from build123d import *

# Parameters (mm, degrees)
SALIENTE_EXTRUIR1_DEPTH = 15.875
REDONDEO1_R             = 15.875
CORTAR_EXTRUIR1_REACH   = 48.084
CROQUIS2_R              = 9.525
CROQUIS3_R              = 12.7
CORTAR_EXTRUIR2_DEPTH   = 47.084243503
CROQUIS4_R              = 3.2639
CROQUIS4_R_2            = 2.4892
CORTAR_EXTRUIR3_DEPTH   = 47.084243503
REDONDEO2_R             = 2.54
REDONDEO3_R             = 1.27


with BuildPart() as part:
    # Croquis1 → Saliente-Extruir1 (new body)
    with BuildSketch(Plane.XY):
        Polygon((30.48, 0), (-30.48, 0), (-30.48, 6.35), (12.046472996, 38.277805334), (30.48, 6.35), align=None)
    extrude(amount=SALIENTE_EXTRUIR1_DEPTH)

    # Redondeo1
    redondeo1_edges = [part.edges().sort_by_distance(p)[0] for p in [
        (12.046472996, 38.277805334, 7.9375),
    ]]
    fillet(redondeo1_edges, radius=REDONDEO1_R)

    # Croquis2 → Cortar-Extruir1 (cut, up to next)
    with BuildSketch(Plane.XY.offset(15.875), mode=Mode.PRIVATE) as cortar_extruir1_sk1:
        with Locations((7.254003, 16.09860686)):
            Circle(CROQUIS2_R)
    cortar_extruir1_tool1 = extrude(cortar_extruir1_sk1.sketch, amount=-CORTAR_EXTRUIR1_REACH, mode=Mode.PRIVATE) & part.part
    add(cortar_extruir1_tool1.solids().sort_by_distance((7.254003, 16.098607, 15.875))[0], mode=Mode.SUBTRACT)

    # Croquis3 → Cortar-Extruir2 (cut, through all)
    with BuildSketch(Plane.XY.offset(15.875)):
        with Locations((7.254003, 16.09860686)):
            Circle(CROQUIS3_R)
    extrude(amount=-CORTAR_EXTRUIR2_DEPTH, mode=Mode.SUBTRACT)

    # Croquis4 → Cortar-Extruir3 (cut, through all)
    with BuildSketch(Plane.XZ):
        with Locations((-23.8125, 11.43)):
            Circle(CROQUIS4_R)
        with Locations(Location((23.8125, 11.43, 0), (0, 0, 210.56660833))):
            Circle(CROQUIS4_R)
        with Locations((7.254003, 9.525)):
            Circle(CROQUIS4_R_2)
    extrude(amount=-CORTAR_EXTRUIR3_DEPTH, mode=Mode.SUBTRACT)

    # Redondeo2
    redondeo2_edges = [part.edges().sort_by_distance(p)[0] for p in [
        (-30.48, 6.35, 7.9375),
        (30.48, 6.35, 7.9375),
    ]]
    fillet(redondeo2_edges, radius=REDONDEO2_R)

    # Redondeo3
    redondeo3_edges = [part.edges().sort_by_distance(p)[0] for p in [
        (30.48, 0, 7.9375),
        (-30.48, 0, 7.9375),
    ]]
    fillet(redondeo3_edges, radius=REDONDEO3_R)


solid = part.part
Model file for the job. Use its own axes, mm. Round coordinates to 2 decimals unless told otherwise and drop trailing zeros. Loops run counter-clockwise (first coordinate to the right, second up) from the corner with the lowest first, then second, coordinate; pieces in that order, holes last. Notation, with made-up numbers: (26.25, 45) - (68.25, 45) arc R13 cw to (68.25, 54) - close; hole circle Ø11 at (86.25, 61.25). An arc over 180 degrees is marked (long way). Write each question's results on one line, items separated by ' | '.
(1) Wall check: L1, parallel to Y at x = 7, z = 1; L2, parallel to X at y = 24, z = 7.25; L3, parallel to X at y = 24.5, z = 3.5. Give the ranges that are in metal, low to high.
Answer below:
L1: y = 0 to 3.4, 28.8 to 30.7 | L2: x = -6.97 to -2.69, 17.2 to 20.21 | L3: x = -6.3 to -2.27, 16.78 to 19.84
(2) Saw through at D-D, the plane z = 1. List the corners of the cut face in (x, y) (3 decimals).
Answer below:
outline: (-30.48, 1.27) arc R1.27 ccw to (-29.21, 0) - (29.21, 0) arc R1.27 ccw to (30.48, 1.27) - (30.48, 5.669) arc R2.54 ccw to (30.14, 6.939) - (21.002, 22.766) arc R15.875 ccw to (-2.277, 27.524) - (-29.465, 7.112) arc R2.54 ccw to (-30.48, 5.081) - close; hole circle Ø25.4 at (7.254, 16.099)
(3) Saw through at A-A, the plane x = -25. List the corners of the cut face in (y, z) (3 decimals), then the cut area to 3 significant figures.
Answer below:
outline: (0, 0) - (10.464, 0) - (10.464, 8.39) - (0, 8.39) - close; (0, 14.47) - (10.464, 14.47) - (10.464, 15.875) - (0, 15.875) - close | area: 102 mm^2
(4) Pin check, flat tips, straight feed: pin 1 (7.5 mm diameter, centred on x = -23.81, z = 11.43, fed in from +Y); pin 2 (8 mm diameter, centred on y = 15, z = 3, fed in from +X); pin 3 (8 mm diameter, centred on x = 15.5, z = 9, fed in from +Y); pin 4 (4 mm diameter, centred on x = 7.25, z = 9.52, fed in from +Y). Stop position of each tip, or through.
Answer below:
pin 1: stops at y = 14.17 | pin 2: stops at x = 27.8 | pin 3: stops at y = 30.13 | pin 4: passes through
(5) Saw through at B-B, the plane z = 8.75. List the corners of the cut face in (x, y) (3 decimals).
Answer below:
outline: (-30.48, 1.27) arc R1.27 ccw to (-29.21, 0) - (-25.675, 0) - (-25.675, 9.957) - (-29.465, 7.112) arc R2.54 ccw to (-30.48, 5.081) - close; (-21.95, 0) - (4.889, 0) - (4.889, 3.621) arc R12.7 cw to (4.889, 28.576) - (4.889, 30.526) arc R15.875 ccw to (-2.277, 27.524) - (-21.95, 12.754) - close; (9.619, 0) - (21.95, 0) - (21.95, 21.125) - (21.002, 22.766) arc R15.875 ccw to (9.619, 30.526) - (9.619, 28.576) arc R12.7 cw to (9.619, 3.621) - close; (25.675, 0) - (29.21, 0) arc R1.27 ccw to (30.48, 1.27) - (30.48, 5.669) arc R2.54 ccw to (30.14, 6.939) - (25.675, 14.672) - close
(6) Mould opens along X. For faces 1 (the cylindrical face through (4.5, 3.7, 8)), 2 (the flat face through (30.48, 4, 8)), 3 (the flat face through (0, 5, 0)) say: released by +X, released by -X, zero draft, split by the parting line, or undercut.
Answer below:
face 1: undercut | face 2: released by +X | face 3: zero draft
(7) Saw through at C-C, the plane y = 2.5. List the corners of the cut face in (x, z) (1 decimal).
Answer below:
outline: (-30.5, 0) - (30.5, 0) - (30.5, 15.9) - (-30.5, 15.9) - close; hole circle Ø6.5 at (-23.8, 11.4); hole circle Ø5 at (7.3, 9.5); hole circle Ø6.5 at (23.8, 11.4)
